Part model, mm, in its own coordinate system. A direction names the side the tool comes from. Round coordinates to 2 decimals unless told otherwise and drop trailing zeros. Loops run counter-clockwise (first coordinate to the right, second up) from the corner with the lowest first, then second, coordinate; pieces in that order, holes last. Notation, with made-up numbers: (65, 23) - (86, 23) arc R9 ccw to (86, 40) - close; hole circle Ø4 at (-1, 57.5). An arc over 180 degrees is marked (long way). Put each result on its own line as item: value.
from build123d import *

# Parameters (mm, degrees)
ESBO_O1_W                = 48
ESBO_O1_H                = 29
ESBO_O1_R                = 1.65
RESSALTO_EXTRUS_O1_DEPTH = 12
CORTE_EXTRUS_O3_START    = 1.5
ESBO_O2_R                = 0.6
CORTE_EXTRUS_O3_DEPTH    = 7
ESBO_O3_R                = 1.65
CORTE_EXTRUS_O4_DEPTH    = 16
CORTE_EXTRUS_O5_DEPTH    = 2
ESBO_O5_W                = 3
ESBO_O5_H                = 5.5
CORTE_EXTRUS_O6_DEPTH    = 7
ESBO_O6_R                = 1.65
CORTE_EXTRUS_O7_DEPTH    = 13
ESBO_O7_R                = 3.4
CORTE_EXTRUS_O9_DEPTH    = 3


with BuildPart() as part:
    # Esboço1 → Ressalto-extrusão1 (new body)
    with BuildSketch(Plane.XY):
        Rectangle(ESBO_O1_W, ESBO_O1_H)
        with Locations((-21, 11)):
            Circle(ESBO_O1_R, mode=Mode.SUBTRACT)
        with Locations((-21, -11)):
            Circle(ESBO_O1_R, mode=Mode.SUBTRACT)
        with Locations((21, -11)):
            Circle(ESBO_O1_R, mode=Mode.SUBTRACT)
        with Locations((21, 11)):
            Circle(ESBO_O1_R, mode=Mode.SUBTRACT)
    extrude(amount=RESSALTO_EXTRUS_O1_DEPTH)

    # Esboço2 → Corte-extrusão3 (cut)
    with BuildSketch(Plane(origin=(0, 0, 0), x_dir=(1, 0, 0), z_dir=(0, 1, 0)).offset(CORTE_EXTRUS_O3_START)):
        with Locations((-23, 0)):
            Circle(ESBO_O2_R)
        with Locations((-21, 0)):
            Circle(ESBO_O2_R)
        with Locations((-19, 0)):
            Circle(ESBO_O2_R)
        with Locations((19, 0)):
            Circle(ESBO_O2_R)
        with Locations((21, 0)):
            Circle(ESBO_O2_R)
        with Locations((23, 0)):
            Circle(ESBO_O2_R)
        with BuildLine():
            Line((-24, -9), (-8, -9))
            ThreePointArc((-8, -9), (-4.818019485, -7.681980515), (-3.5, -4.5))
            Line((-3.5, -4.5), (-3.5, 0))
            Line((-3.5, 0), (-18, 0))
            Line((-18, 0), (-18, -7.5))
            Line((-18, -7.5), (-24, -7.5))
            Line((-24, -7.5), (-24, -9))
        make_face()
        with BuildLine():
            Line((24, -7.5), (24, -9))
            Line((24, -9), (8, -9))
            ThreePointArc((8, -9), (4.818019485, -7.681980515), (3.5, -4.5))
            Line((3.5, -4.5), (3.5, 0))
            Line((3.5, 0), (18, 0))
            Line((18, 0), (18, -7.5))
            Line((18, -7.5), (24, -7.5))
        make_face()
    corte_extrus_o3 = extrude(amount=CORTE_EXTRUS_O3_DEPTH, mode=Mode.SUBTRACT)

    # Espelhar1: Corte-extrusão3 across plane
    add(corte_extrus_o3.mirror(Plane.ZX), mode=Mode.SUBTRACT)

    # Esboço3 → Corte-extrusão4 (cut)
    with BuildSketch(Plane(origin=(24, 0, 0), x_dir=(0, 0, -1), z_dir=(1, 0, 0))):
        with Locations((-3.75, 5)):
            Circle(ESBO_O3_R)
        with Locations((-3.75, -5)):
            Circle(ESBO_O3_R)
    corte_extrus_o4 = extrude(amount=-CORTE_EXTRUS_O4_DEPTH, mode=Mode.SUBTRACT)

    # Esboço4 → Corte-extrusão5 (cut)
    with BuildSketch(Plane.ZY.offset(-18)):
        Polygon((6.925426481, 5), (5.33771324, 7.75), (2.16228676, 7.75), (0.574573519, 5), (2.16228676, 2.25), (5.33771324, 2.25), align=None)
        Polygon((6.925426481, -5), (5.33771324, -2.25), (2.16228676, -2.25), (0.574573519, -5), (2.16228676, -7.75), (5.33771324, -7.75), align=None)
    corte_extrus_o5 = extrude(amount=-CORTE_EXTRUS_O5_DEPTH, mode=Mode.SUBTRACT)

    # Esboço5 → Corte-extrusão6 (cut)
    with BuildSketch(Plane(origin=(24, 0, 0), x_dir=(0, 0, -1), z_dir=(1, 0, 0))):
        with Locations((-5, 0)):
            Rectangle(ESBO_O5_W, ESBO_O5_H)
        with Locations((-5, 11)):
            Rectangle(ESBO_O5_W, ESBO_O5_H)
        with Locations((-5, -11)):
            Rectangle(ESBO_O5_W, ESBO_O5_H)
    corte_extrus_o6 = extrude(amount=-CORTE_EXTRUS_O6_DEPTH, mode=Mode.SUBTRACT)

    # Esboço6 → Corte-extrusão7 (cut, through all)
    with BuildSketch(Plane(origin=(0, 0, 0), x_dir=(-1, 0, 0), z_dir=(0, 0, -1))):
        with Locations((-21, 0)):
            Circle(ESBO_O6_R)
        with Locations((21, 0)):
            Circle(ESBO_O6_R)
        Circle(ESBO_O6_R)
        with Locations((0, 11)):
            Circle(ESBO_O6_R)
        with Locations((0, -11)):
            Circle(ESBO_O6_R)
    extrude(amount=-CORTE_EXTRUS_O7_DEPTH, mode=Mode.SUBTRACT)

    # Espelhar2: Corte-extrusão4, Corte-extrusão5, Corte-extrusão6 across plane
    add(corte_extrus_o4.mirror(Plane(origin=(0, 0, 0), x_dir=(0, 0, 1), z_dir=(1, 0, 0))), mode=Mode.SUBTRACT)
    add(corte_extrus_o5.mirror(Plane(origin=(0, 0, 0), x_dir=(0, 0, 1), z_dir=(1, 0, 0))), mode=Mode.SUBTRACT)
    add(corte_extrus_o6.mirror(Plane(origin=(0, 0, 0), x_dir=(0, 0, 1), z_dir=(1, 0, 0))), mode=Mode.SUBTRACT)

    # Esboço7 → Corte-extrusão9 (cut)
    with BuildSketch(Plane(origin=(0, 0, 0), x_dir=(-1, 0, 0), z_dir=(0, 0, -1))):
        with Locations((0, 11)):
            Circle(ESBO_O7_R)
        Circle(ESBO_O7_R)
        with Locations((0, -11)):
            Circle(ESBO_O7_R)
    extrude(amount=-CORTE_EXTRUS_O9_DEPTH, mode=Mode.SUBTRACT)


solid = part.part
1. Two-plate mould, pull along Z, no slides. Class faces 5 (the flat face through (19, 11, 6.5)), 6 (the cylindrical face through (-22.31, -12, 9.21)), 7 (the cylindrical face through (-21, 5, 0.6)): pulls with the +Z half, pulls with the -Z half, needs draft (parallel to the pull), parting line crosses it, or undercut.
A:
face 5: undercut
face 6: needs draft
face 7: pulls with the -Z half
2. Tool access for faces 1 (the flat face through (22, -2.75, 5)), 2 (the cylindrical face through (4.853, -4.951, 7.717)), 3 (the cylindrical face through (-22.03, 4, 5.06)), 4 (the flat face through (19, -7.75, 4)): list every direction of +Z, -Z, +X, -X, +Y, -Y with a clear straight run to the whole face (end or side of a thin tool).
A:
face 1: +X
face 2: -Z
face 3: -X
face 4: none
3. Probe line 1 along Y through (x, z) = (5.5, 7); line 2 along X through (y, z) = (5.75, 1.5); line 3 along Y through (x, z) = (-21.7, 3.75). List the from-to ranges inside material, lowest first. Write a range as [from, to].
A:
line 1: y = [-14.5, -8.5], [-1.5, 1.5], [8.5, 14.5]
line 2: x = [-24, -20], [-3.5, 3.5], [20, 24]
line 3: y = [-14.5, -13.75], [-8.25, -6.65], [-3.35, -2.75], [2.75, 3.35], [6.65, 8.25], [13.75, 14.5]
4. Band-saw the part on A-A (z = 10.25). Give the number of separate pieces and of enclosed holes in the cut face, plus the area to 3 significant figures.
A:
separate pieces: 1
enclosed holes: 9
area: 1,320 mm²
5. Band-saw the part on C-C (x = -10.5). List the corners of the cut face in (y, z).
A:
outline: (-14.5, 0) - (-8.5, 0) - (-8.5, 9) - (-1.5, 9) - (-1.5, 0) - (1.5, 0) - (1.5, 9) - (8.5, 9) - (8.5, 0) - (14.5, 0) - (14.5, 12) - (-14.5, 12) - close
